Here's how the part is built. I have some questions about the finished solid (model axes, mm). Face numbers are marked on the shaded views. Give positions to 0.01 mm unless a question says otherwise; leave off trailing zeros. Order: outer loops, then holes, each group sorted by start corner. A loop starts at its lowest first (then second) coordinate and runs counter-clockwise, first axis right, second up.
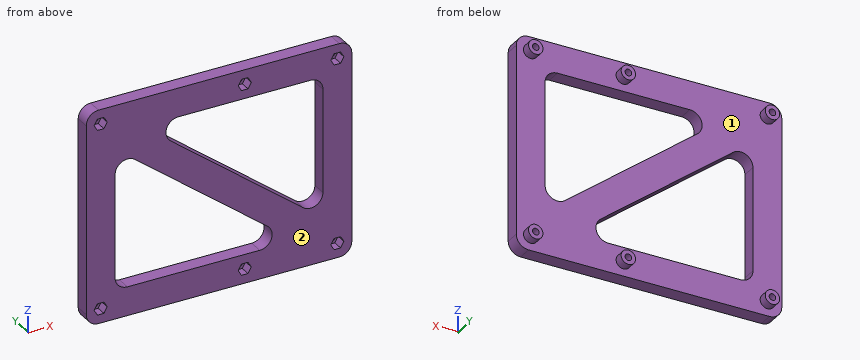
from build123d import *

# Parameters (mm, degrees)
SKETCH1_W           = 129
SKETCH1_H           = 104
SKETCH1_R           = 3.5
BOSS_EXTRUDE1_DEPTH = 7
FILLET1_R           = 6
SKETCH1_3_R         = 3.5
SKETCH1_3_R_2       = 1.6
BOSS_EXTRUDE2_DEPTH = 11.4
SKETCH2_R           = 1.6
CUT_EXTRUDE1_DEPTH  = 5


with BuildPart() as part:
    # Sketch1 → Boss-Extrude1 (new body)
    with BuildSketch(Plane(origin=(0, 0, 0), x_dir=(1, 0, 0), z_dir=(0, 1, 0))):
        Rectangle(SKETCH1_W, SKETCH1_H)
        with Locations((57.5, -45)):
            Circle(SKETCH1_R, mode=Mode.SUBTRACT)
        with Locations((12.5, -45)):
            Circle(SKETCH1_R, mode=Mode.SUBTRACT)
        with Locations((-57.5, -45)):
            Circle(SKETCH1_R, mode=Mode.SUBTRACT)
        with Locations((57.5, 45)):
            Circle(SKETCH1_R, mode=Mode.SUBTRACT)
        with Locations((12.5, 45)):
            Circle(SKETCH1_R, mode=Mode.SUBTRACT)
        with Locations((-57.5, 45)):
            Circle(SKETCH1_R, mode=Mode.SUBTRACT)
        Polygon((37.197602993, 38), (-50.5, 38), (-50.5, -30.63290669), align=None, mode=Mode.SUBTRACT)
        Polygon((50.5, 30.63290669), (-37.197602993, -38), (50.5, -38), align=None, mode=Mode.SUBTRACT)
    extrude(amount=BOSS_EXTRUDE1_DEPTH)

    # Fillet1
    fillet1_edges = [part.edges().sort_by_distance(p)[0] for p in [
        (-64.5, 3.5, 52),
        (-64.5, 3.5, -52),
        (64.5, 3.5, -52),
        (64.5, 3.5, 52),
        (-37.197602993, 3.5, 38),
        (50.5, 3.5, 38),
        (50.5, 3.5, -30.63290669),
        (-50.5, 3.5, -38),
        (-50.5, 3.5, 30.63290669),
        (37.197602993, 3.5, -38),
    ]]
    fillet(fillet1_edges, radius=FILLET1_R)

    # Sketch1_3 → Boss-Extrude2 (add)
    with BuildSketch(Plane(origin=(0, 0, 0), x_dir=(1, 0, 0), z_dir=(0, 1, 0))):
        with Locations((-57.5, -45)):
            Circle(SKETCH1_3_R)
        with Locations((-57.5, -45)):
            Circle(SKETCH1_3_R_2, mode=Mode.SUBTRACT)
        with Locations((-57.5, 45)):
            Circle(SKETCH1_3_R)
        with Locations((-57.5, 45)):
            Circle(SKETCH1_3_R_2, mode=Mode.SUBTRACT)
        with Locations((12.5, 45)):
            Circle(SKETCH1_3_R)
        with Locations((12.5, 45)):
            Circle(SKETCH1_3_R_2, mode=Mode.SUBTRACT)
        with Locations((57.5, 45)):
            Circle(SKETCH1_3_R)
        with Locations((57.5, 45)):
            Circle(SKETCH1_3_R_2, mode=Mode.SUBTRACT)
        with Locations((12.5, -45)):
            Circle(SKETCH1_3_R)
        with Locations((12.5, -45)):
            Circle(SKETCH1_3_R_2, mode=Mode.SUBTRACT)
        with Locations((57.5, -45)):
            Circle(SKETCH1_3_R)
        with Locations((57.5, -45)):
            Circle(SKETCH1_3_R_2, mode=Mode.SUBTRACT)
    extrude(amount=BOSS_EXTRUDE2_DEPTH)

    # Sketch2 → Cut-Extrude1 (cut)
    with BuildSketch(Plane.XZ):
        Polygon((-54.324573519, 45), (-55.91228676, 47.75), (-59.08771324, 47.75), (-60.675426481, 45), (-59.08771324, 42.25), (-55.91228676, 42.25), align=None)
        with Locations((-57.5, 45)):
            Circle(SKETCH2_R, mode=Mode.SUBTRACT)
        Polygon((15.675426481, 45), (14.08771324, 47.75), (10.91228676, 47.75), (9.324573519, 45), (10.91228676, 42.25), (14.08771324, 42.25), align=None)
        with Locations((12.5, 45)):
            Circle(SKETCH2_R, mode=Mode.SUBTRACT)
        Polygon((60.675426481, 45), (59.08771324, 47.75), (55.91228676, 47.75), (54.324573519, 45), (55.91228676, 42.25), (59.08771324, 42.25), align=None)
        with Locations((57.5, 45)):
            Circle(SKETCH2_R, mode=Mode.SUBTRACT)
        Polygon((-54.324573519, -45), (-55.91228676, -42.25), (-59.08771324, -42.25), (-60.675426481, -45), (-59.08771324, -47.75), (-55.91228676, -47.75), align=None)
        with Locations((-57.5, -45)):
            Circle(SKETCH2_R, mode=Mode.SUBTRACT)
        Polygon((15.675426481, -45), (14.08771324, -42.25), (10.91228676, -42.25), (9.324573519, -45), (10.91228676, -47.75), (14.08771324, -47.75), align=None)
        with Locations((12.5, -45)):
            Circle(SKETCH2_R, mode=Mode.SUBTRACT)
        Polygon((60.675426481, -45), (59.08771324, -42.25), (55.91228676, -42.25), (54.324573519, -45), (55.91228676, -47.75), (59.08771324, -47.75), align=None)
        with Locations((57.5, -45)):
            Circle(SKETCH2_R, mode=Mode.SUBTRACT)
    extrude(amount=-CUT_EXTRUDE1_DEPTH, mode=Mode.SUBTRACT)


solid = part.part
Q1. I need wall thicknesses on L1, parallel to Z at x = 12.5, y = 8.75; L2, parallel to X at y = 9.75, z = 45; L3, parallel to Z at x = -57.5, y = 6.75. Which ranges of each line are inside material? Lowest first, please.
Filled sheet:
L1: z = -48.5 to -46.6, -43.4 to -41.5, 41.5 to 43.4, 46.6 to 48.5
L2: x = -61 to -59.1, -55.9 to -54, 9 to 10.9, 14.1 to 16, 54 to 55.9, 59.1 to 61
L3: z = -52 to -46.6, -43.4 to 43.4, 46.6 to 52
Q2. If we section it at C-C on z = -30: List the corners of the cut face in (x, y) for me, plus the area to 3 significant figures.
Filled sheet:
outline: (-64.5, 0) - (-50.5, 0) - (-50.5, 7) - (-64.5, 7) - close; (25.45, 0) - (64.5, 0) - (64.5, 7) - (25.45, 7) - close
area: 371 mm2
Q3. If we section it at B-B on x = -32: List the corners of the cut face in (y, z) for me, plus the area to 3 significant figures.
Filled sheet:
outline: (0, -52) - (7, -52) - (7, -38) - (0, -38) - close; (0, 16.15) - (7, 16.15) - (7, 52) - (0, 52) - close
area: 349 mm2
Q4. If we section it at D-D on x = -9: List the corners of the cut face in (y, z) for me, plus the area to 3 significant figures.
Filled sheet:
outline: (0, -52) - (7, -52) - (7, -38) - (0, -38) - close; (0, -1.85) - (7, -1.85) - (7, 15.93) - (0, 15.93) - close; (0, 38) - (7, 38) - (7, 52) - (0, 52) - close
area: 320 mm2
Q5. If we section it at A-A on y = 9.75: Give the number of separate pieces and of enclosed holes in the cut face, plus the area to 3 significant figures.
Filled sheet:
separate pieces: 6
enclosed holes: 6
area: 183 mm2
Q6. Thinking about a two-plate mould opening in Z: for the marked faces 1 and 2, which applies, released by +Z, released by -Z, zero draft, split by the parting line, or undercut?
Filled sheet:
face 1: undercut
face 2: zero draft
Q7. I'm going to push flat-ended pins straight in: P1, Ø6, axis at x = -58.5, z = -44, coming from the -Y side; P2, Ø1.6, axis at x = 58.5, z = 46, coming from the -Y side; P3, Ø12, axis at x = 30, z = -4, coming from the +Y side. Where does each tip first touch, or does it pass through?
Filled sheet:
P1: stops at y = 0
P2: stops at y = 5
P3: passes through
